```python
from build123d import *

# Parameters (mm, degrees)
F0_W     = 137.691636
F0_H     = 81.126414
F1_DEPTH = 76.2
F2_T     = -7.62
F3_W     = 56.93736
F3_H     = 51.178044
F4_DEPTH = 81.127414
F5_R     = 9.811044
F6_DEPTH = 137.692636


with BuildPart() as f1:
    # F0 (on Top) → F1 (new body)
    with BuildSketch(Plane.XY):
        with Locations((2.791045, 0)):
            Rectangle(F0_W, F0_H)
    extrude(amount=F1_DEPTH)

    # F2
    f2_openings = [f1.faces().sort_by_distance(p)[0] for p in [
        (2.791045, 0, 76.2),
        (2.791045, 0, 0),
    ]]
    offset(amount=F2_T, openings=f2_openings)

    # F3 (on face) → F4 (cut, through all)
    with BuildSketch(Plane.XZ.offset(40.563207)):
        with Locations((0, 76.2)):
            Rectangle(F3_W, F3_H)
    extrude(amount=-F4_DEPTH, mode=Mode.SUBTRACT)

    # F5 (on face) → F6 (cut, through all)
    with BuildSketch(Plane.YZ.offset(71.636863)):
        with Locations((0, 38.1)):
            Circle(F5_R)
    extrude(amount=-F6_DEPTH, mode=Mode.SUBTRACT)


solid = f1.part
```
Here's how the part is built. I have some questions about the finished solid (model axes, mm). A direction names the side the tool comes from. Coordinates: 2 decimals unless noted, no trailing zeros. Write each loop counter-clockwise with the first axis right and the second up, starting at its lowest first coordinate (ties: lowest second). Pieces come first, ordered by that corner, then holes. Notation, with made-up numbers: M -7.75,-36.75 L 4.25,-36.75 A15 cw 4.25,-12.75 Z; hole C -25,-3 d9. An arc over 180 degrees is marked long. Answer as CSV lines item,"result". Start each with the question number.
Q1. Suppose I cut it at B-B, the plane z = 38.1. List the corners of the cut face in (x, y) for me.
Q2. Will these pins go through, and if not, where does the flat tip stop? pin 1 Ø10 at (x, y) = (56.5, -19) entering from +Z; pin 2 Ø8.5 at (x, y) = (9, -36.5) entering from +Z.
Q3. Suppose I cut it at C-C, the plane y = 0. List the corners of the cut face in (x, z) for me.
Q4. If we mould it in two halves opening along X, with no side actions, what happens to faces 1 (the flat face through (64.017, -8, 46)), 2 (the flat face through (71.637, -10, 46)), 3 (the flat face through (69, 1, 76.2))? For each: pulls with the +X half, pulls with the -X half, needs draft (parallel to the pull), parting line crosses it, or undercut.
Q5. Suppose I cut it at D-D, the plane x = -36. List the corners of the cut face in (y, z) for me, then the cut area to 3 significant figures.
Q6. For faces 4 (the flat face through (-28.469, -37, 63)), 5 (the flat face through (-58.435, -8, 46)), 6 (the flat face through (-66.055, -10, 46)), which set-ups out of +Z, -Z, +X, -X, +Y, -Y let a thin tool reach every point of the face, with its end or its side?
Q7. Suppose I cut it at A-A, the plane y = -16. List the corners of the cut face in (x, z) for me, then the cut area to 3 significant figures.
Q8. I need wall thicknesses on probe 1 along X at (y, z) = (-21, 4); probe 2 along X at (y, z) = (36, 71); probe 3 along Y at (x, z) = (-26, 27). Which ranges of each line are inside material? Lowest first, please. Write a range as [from, to].
Entries:
1,outline,"M -66.05,-40.56 L 71.64,-40.56 L 71.64,-9.81 L 64.02,-9.81 L 64.02,-32.94 L -58.43,-32.94 L -58.43,-9.81 L -66.05,-9.81 Z; M -66.05,9.81 L -58.43,9.81 L -58.43,32.94 L 64.02,32.94 L 64.02,9.81 L 71.64,9.81 L 71.64,40.56 L -66.05,40.56 Z"
2,pin 1,"passes through"
2,pin 2,"stops at z = 50.61"
3,outline,"M -66.05,0 L -58.43,0 L -58.43,28.29 L -66.05,28.29 Z; M -66.05,47.91 L -58.43,47.91 L -58.43,76.2 L -66.05,76.2 Z; M 64.02,0 L 71.64,0 L 71.64,28.29 L 64.02,28.29 Z; M 64.02,47.91 L 71.64,47.91 L 71.64,76.2 L 64.02,76.2 Z"
4,face 1,"undercut"
4,face 2,"pulls with the +X half"
4,face 3,"needs draft"
5,outline,"M -40.56,0 L -32.94,0 L -32.94,76.2 L -40.56,76.2 Z; M 32.94,0 L 40.56,0 L 40.56,76.2 L 32.94,76.2 Z"
5,area,"1,160 mm²"
6,face 4,"+Z, +Y, -Y"
6,face 5,"+Z, -Z"
6,face 6,"+Z, -Z, -X, +Y, -Y"
7,outline,"M -66.05,0 L -58.43,0 L -58.43,76.2 L -66.05,76.2 Z; M 64.02,0 L 71.64,0 L 71.64,76.2 L 64.02,76.2 Z"
7,area,"1,160 mm²"
8,probe 1,"x = [-66.05, -58.43], [64.02, 71.64]"
8,probe 2,"x = [-66.05, -28.47], [28.47, 71.64]"
8,probe 3,"y = [-40.56, -32.94], [32.94, 40.56]"
